The model under review builds one solid part; all positions refer to its coordinate system, in mm. A direction names the side the tool comes from. Give positions to 0.01 mm unless a question says otherwise; leave off trailing zeros. Loops run counter-clockwise (first coordinate to the right, second up) from the corner with the lowest first, then second, coordinate; pieces in that order, holes last. Notation, with made-up numbers: M 69,84 L 78,84 A32 cw 78,123 Z; hole C 17,27 d10. An arc over 180 degrees is marked long. Put each result on its own line as item: value. Start each with the question number.
```python
from build123d import *

# Parameters (mm, degrees)
BOSS_EXTRUDE1_DEPTH = 2
CHAMFER1_SIZE       = 2


with BuildPart() as part:
    # Sketch1 → Boss-Extrude1 (new body)
    with BuildSketch(Plane(origin=(0, 0, 0), x_dir=(1, 0, 0), z_dir=(0, 1, 0))):
        Polygon((0, -50), (0, 0), (0, 2), (-40, 2), (-70, -2), (-100, -2), (-92, -50), align=None)
    extrude(amount=BOSS_EXTRUDE1_DEPTH)

    # Chamfer1
    chamfer1_edges = [part.edges().sort_by_distance(p)[0] for p in [
        (-46, 0, 50),
    ]]
    chamfer(chamfer1_edges, length=CHAMFER1_SIZE - 0.0001)  # a hair under: the kernel refuses the full size


solid = part.part
```
Item 1: Consider section B-B, the plane y = 0.6. Write out the cut boundary in (x, z), plus the area to 3 significant figures.
Item 2: Consider section C-C, the plane z = 35. Write out the cut boundary in (x, y), plus the area to 3 significant figures.
Item 3: To check wall thickness, follow L1, parallel to Z at x = -92, y = 0.5; L2, parallel to X at y = 0.7, z = 25; L3, parallel to X at y = 1, z = 32. State the ranges of each line that lie inside material, in increasing order. Write a range as [from, to].
Item 4: Clearance check with a flat-ended pin moving along its axis: pin 1 Ø1 at (x, y) = (-29, 1) entering from +Z. State where the tip first meets the part, or that it passes through.
Item 5: Tool access review of faces 1 (the flat face through (0, 1, 24)), 2 (the flat face through (-85, 1, 2)): name each direction out of +Z, -Z, +X, -X, +Y, -Y from which nothing blocks a thin tool from reaching the whole face with its end or side.
Report:
1. outline: M -100,2 L -70,2 L -40,-2 L 0,-2 L 0,48.6 L -92.23,48.6 Z
1. area: 4,700 mm²
2. outline: M -94.5,0 L 0,0 L 0,2 L -94.5,2 Z
2. area: 189 mm²
3. L1: [2, 48.5]
3. L2: [-96.17, 0]
3. L3: [-95, 0]
4. pin 1: z = 49.5
5. face 1: +Z, -Z, +X, +Y, -Y
5. face 2: -Z, -X, +Y, -Y
